from build123d import *

# Parameters (mm, degrees)
EXTRUDE_1_DEPTH     = 50
SKETCH_2_R          = 1.75
CUT_EXTRUDE_1_DEPTH = 53.252813616


with BuildPart() as part:
    # 草图1 → 凸台-拉伸1 (new body)
    with BuildSketch(Plane(origin=(0, 0, 0), x_dir=(1, 0, 0), z_dir=(0, 1, 0))):
        with BuildLine():
            Line((-8.053167235, 9.292821463), (1.946832765, 9.292821463))
            ThreePointArc((1.946832765, 9.292821463), (3.361046328, 8.707035025), (3.946832765, 7.292821463))
            Line((3.946832765, 7.292821463), (3.946832765, -4.777178537))
            ThreePointArc((3.946832765, -4.777178537), (3.361046328, -6.191392099), (1.946832765, -6.777178537))
            Line((1.946832765, -6.777178537), (-8.053167235, -6.777178537))
            Line((-8.053167235, -6.777178537), (-8.053167235, -3.992178537))
            Line((-8.053167235, -3.992178537), (1.946832765, -3.992178537))
            Line((1.946832765, -3.992178537), (1.946832765, 6.507821463))
            Line((1.946832765, 6.507821463), (-8.053167235, 6.507821463))
            Line((-8.053167235, 6.507821463), (-8.053167235, 9.292821463))
        make_face()
    extrude(amount=EXTRUDE_1_DEPTH)

    # 草图2 → 切除-拉伸1 (cut, through all)
    with BuildSketch(Plane(origin=(3.946832765, 0, 0), x_dir=(0, 0, -1), z_dir=(1, 0, 0))):
        with Locations((1.257821463, 45)):
            Circle(SKETCH_2_R)
        with Locations((1.257821463, 5)):
            Circle(SKETCH_2_R)
    extrude(amount=-CUT_EXTRUDE_1_DEPTH, mode=Mode.SUBTRACT)


solid = part.part
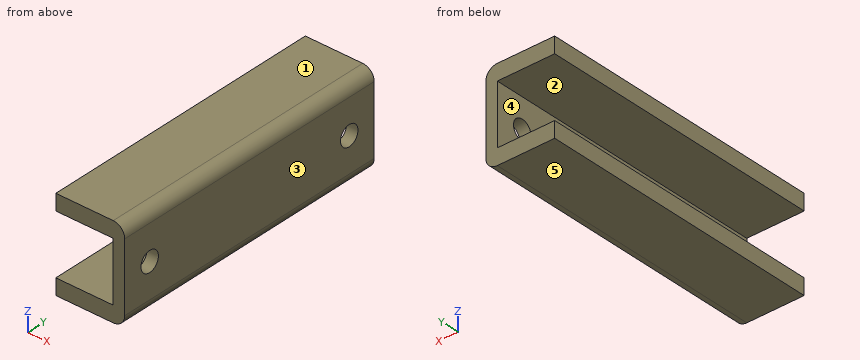
Read the model definition and answer for the solid it produces. Units are mm, in the model's axes. Face numbers are marked on the shaded views. A direction names the side the tool comes from. Round coordinates to 2 decimals unless told otherwise and drop trailing zeros. Write each loop counter-clockwise with the first axis right and the second up, starting at its lowest first coordinate (ties: lowest second). Pieces come first, ordered by that corner, then holes.
1. The part is cut by section A-A, the plane x = -1. Determine the outline of the cut face in (y, z).
2. The part is cut by section B-B, the plane y = 5. Determine the outline of the cut face in (x, z).
3. The part is cut by section D-D, the plane x = 2.75. Determine the outline of the cut face in (y, z).
4. Determine the mould class of the marked faces 1, 2 and 3 for opening direction Z: pulls with the +Z half, pulls with the -Z half, needs draft (parallel to the pull), parting line crosses it, or undercut.
5. Which of the six approach directions +Z, -Z, +X, -X, +Y, -Y give full straight-line access (tool end or side, diameter ignored) to the marked faces 4 and 5?
6. Straight lines are drawn through the part: L1, parallel to Z at x = -4.25, y = 2; L2, parallel to X at y = 14, z = 1.25; L3, parallel to Y at x = 2.25, z = -0.25. For each, find the intervals that lie inside material, in ascending order.
7. The part is cut by section C-C, the plane z = -2.5. Determine the outline of the cut face in (x, y).
8. Given pin 1 Ø3 at (y, z) = (28, -3.5) entering from -X; pin 2 Ø3 at (y, z) = (5, -1.26) entering from -X (3 decimals), each flat-ended and moving along its own axis, determine where each tip first touches the part or whether it passes through.
Values:
1. outline: (0, -9.29) - (50, -9.29) - (50, -6.51) - (0, -6.51) - close; (0, 3.99) - (50, 3.99) - (50, 6.78) - (0, 6.78) - close
2. outline: (-8.05, -9.29) - (1.95, -9.29) arc R2 ccw to (3.95, -7.29) - (3.95, -3.01) - (1.95, -3.01) - (1.95, -6.51) - (-8.05, -6.51) - close; (-8.05, 3.99) - (1.95, 3.99) - (1.95, 0.49) - (3.95, 0.49) - (3.95, 4.78) arc R2 ccw to (1.95, 6.78) - (-8.05, 6.78) - close
3. outline: (0, -9.12) - (50, -9.12) - (50, 6.61) - (0, 6.61) - close; hole circle Ø3.5 at (5, -1.26); hole circle Ø3.5 at (45, -1.26)
4. face 1: pulls with the +Z half
4. face 2: undercut
4. face 3: needs draft
5. face 4: -X, +Y, -Y
5. face 5: -Z, +X, -X, +Y, -Y
6. L1: z = -9.29 to -6.51, 3.99 to 6.78
6. L2: x = 1.95 to 3.95
6. L3: y = 0 to 3.57, 6.43 to 43.57, 46.43 to 50
7. outline: (1.95, 0) - (3.95, 0) - (3.95, 3.77) - (1.95, 3.77) - close; (1.95, 6.23) - (3.95, 6.23) - (3.95, 43.77) - (1.95, 43.77) - close; (1.95, 46.23) - (3.95, 46.23) - (3.95, 50) - (1.95, 50) - close
8. pin 1: stops at x = 1.95
8. pin 2: passes through
